Geometry: final body of the model. Coordinates: model frame, mm. A direction names the side the tool comes from. Give positions to 0.01 mm unless a question says otherwise; leave off trailing zeros. Loops run counter-clockwise (first coordinate to the right, second up) from the corner with the lowest first, then second, coordinate; pieces in that order, holes last.
```python
from build123d import *

# Parameters (mm, degrees)
SKETCH1_R           = 1.5
BOSS_EXTRUDE1_DEPTH = 3
SKETCH2_W           = 40
SKETCH2_H           = 3
CUT_EXTRUDE1_DEPTH  = 3
BOSS_EXTRUDE2_DEPTH = 3
FILLET1_R           = 2
FILLET2_R           = 2


with BuildPart() as part:
    # Sketch1 → Boss-Extrude1 (new body)
    with BuildSketch(Plane(origin=(0, 0, 0), x_dir=(1, 0, 0), z_dir=(0, 1, 0))):
        with BuildLine():
            Line((-19, -20), (19, -20))
            ThreePointArc((19, -20), (20.414213562, -19.414213562), (21, -18))
            Line((21, -18), (21, 18))
            ThreePointArc((21, 18), (20.414213562, 19.414213562), (19, 20))
            Line((19, 20), (-19, 20))
            Line((-19, 20), (-21, 20))
            Line((-21, 20), (-21, 18))
            Line((-21, 18), (-21, -18))
            Line((-21, -18), (-21, -20))
            Line((-21, -20), (-19, -20))
        make_face()
        with Locations(Location((13.5, 15.5, 0), (0, 0, 270))):
            Circle(SKETCH1_R, mode=Mode.SUBTRACT)
        with Locations(Location((-10, 15.5, 0), (0, 0, 270))):
            Circle(SKETCH1_R, mode=Mode.SUBTRACT)
        with Locations(Location((-10, -14.5, 0), (0, 0, 270))):
            Circle(SKETCH1_R, mode=Mode.SUBTRACT)
        with Locations(Location((13.5, -14.5, 0), (0, 0, 270))):
            Circle(SKETCH1_R, mode=Mode.SUBTRACT)
    extrude(amount=BOSS_EXTRUDE1_DEPTH)

    # Sketch2 → Cut-Extrude1 (cut)
    with BuildSketch(Plane.ZY.offset(21)):
        with Locations((0, 1.5)):
            Rectangle(SKETCH2_W, SKETCH2_H)
    extrude(amount=-CUT_EXTRUDE1_DEPTH, mode=Mode.SUBTRACT)

    # Sketch3 → Boss-Extrude2 (add)
    with BuildSketch(Plane.ZY.offset(18)):
        with BuildLine():
            Line((-20, 3), (20, 3))
            Line((20, 3), (20, -23))
            ThreePointArc((20, -23), (0, -43), (-20, -23))
            Line((-20, -23), (-20, 3))
        make_face()
        with BuildLine():
            Line((-6.25, -30.25), (-6.25, -15.75))
            ThreePointArc((-6.25, -15.75), (0, -9.5), (6.25, -15.75))
            Line((6.25, -15.75), (6.25, -30.25))
            ThreePointArc((6.25, -30.25), (0, -36.5), (-6.25, -30.25))
        make_face(mode=Mode.SUBTRACT)
    extrude(amount=BOSS_EXTRUDE2_DEPTH)

    # Fillet1
    fillet1_edges = [part.edges().sort_by_distance(p)[0] for p in [
        (-21, 3, 0),
    ]]
    fillet(fillet1_edges, radius=FILLET1_R)

    # Fillet2
    fillet2_edges = [part.edges().sort_by_distance(p)[0] for p in [
        (-18, 0, 0),
    ]]
    fillet(fillet2_edges, radius=FILLET2_R)


solid = part.part
```
Q1. Pin query (flat end, axial travel): pin 1 Ø6 at (x, z) = (-12.5, 14) entering from -Y; pin 2 Ø1.8 at (x, z) = (-10, -15.5) entering from +Y; pin 3 Ø4 at (y, z) = (-22.5, 8) entering from +X; pin 4 Ø3.5 at (x, y) = (-19.5, -25) entering from -Z. Return the tip coordinate at first contact, or that it passes through.
Q2. Section query A-A, the plane x = 13.5. Return loops of the section in (y, z).
Q3. Material intervals for probe 1 along X at (y, z) = (1.5, 14.5); probe 2 along X at (y, z) = (-4, 4.5); probe 3 along Y at (x, z) = (-10.5, -13.5), sorted ascending.
Q4. Section query D-D, the plane z = -15.5. Return loops of the section in (x, y), and give its area (3 significant figures).
Q5. Section query B-B, the plane z = 0. Return loops of the section in (x, y), and give its area (3 significant figures).
Q6. Reachability of faces 4 (the face through (-19, -43, 0)), 5 (the face through (-18, -22, -9)), 6 (the face through (-19.5, -9.5, -0.1)) from +Z, -Z, +X, -X, +Y, -Y: full face, straight path, thin tool, end or side. Return the list, or none.
Q7. Section query C-C, the plane y = -20. Return loops of the section in (x, z), and give its area (3 significant figures).
Q8. Mould query, pull axis X, two halves, no side actions, for faces 1 (the face through (-19, -23, 6.25)), 2 (the face through (21, 1, 0)), 3 (the face through (-10, 1, -17)). Classes: +X half, -X half, draft (parallel to the pull), parting line (faces both ways), or undercut.
Resolved:
1. pin 1: stops at y = 0
1. pin 2: passes through
1. pin 3: stops at x = -18
1. pin 4: stops at z = -20
2. outline: (0, -20) - (3, -20) - (3, -17) - (0, -17) - close; (0, -14) - (3, -14) - (3, 13) - (0, 13) - close; (0, 16) - (3, 16) - (3, 20) - (0, 20) - close
3. probe 1: x = -20.94 to -11.5, -8.5 to 12, 15 to 21
3. probe 2: x = -21 to -18
3. probe 3: y = 0 to 3
4. outline: (-21, -35.64) - (-18, -35.64) - (-18, -2) arc R2 cw to (-16, 0) - (-11.5, 0) - (-11.5, 3) - (-19, 3) arc R2 ccw to (-21, 1) - close; (-8.5, 0) - (12, 0) - (12, 3) - (-8.5, 3) - close; (15, 0) - (21, 0) - (21, 3) - (15, 3) - close
4. area: 215 mm2
5. outline: (-21, -43) - (-18, -43) - (-18, -36.5) - (-21, -36.5) - close; (-21, -9.5) - (-18, -9.5) - (-18, -2) arc R2 cw to (-16, 0) - (21, 0) - (21, 3) - (-19, 3) arc R2 ccw to (-21, 1) - close
5. area: 174 mm2
6. face 4: +X, -X, -Y
6. face 5: +Z, -Z, +X, -Y
6. face 6: +X, -X
7. outline: (-21, -20) - (-18, -20) - (-18, -6.25) - (-21, -6.25) - close; (-21, 6.25) - (-18, 6.25) - (-18, 20) - (-21, 20) - close
7. area: 82.5 mm2
8. face 1: draft
8. face 2: +X half
8. face 3: undercut
